Geometry check sheet. Reference: the model listing, model coordinates, mm. A direction names the side the tool comes from. Coordinates: 2 decimals unless noted, no trailing zeros. Loops run counter-clockwise (first coordinate to the right, second up) from the corner with the lowest first, then second, coordinate; pieces in that order, holes last. Notation, with made-up numbers: (-13.5, 48) -> (3.5, 48) arc R21 ccw to (3.5, 61) -> close; hole circle Ø8 at (28.25, -28.75). An arc over 180 degrees is marked (long way). Answer as a JSON object with one key per item and string values.
from build123d import *

# Parameters (mm, degrees)
SKETCH1_R           = 0.95
SKETCH1_R_2         = 2
SKETCH1_R_3         = 3
SKETCH1_R_4         = 1.047925013
SKETCH1_R_5         = 0.495
SKETCH1_R_6         = 0.65
BOSS_EXTRUDE1_DEPTH = 17.78
CUT_EXTRUDE1_DEPTH  = 14.78
BOSS_EXTRUDE2_DEPTH = 3
SKETCH4_W           = 10.78
SKETCH4_H           = 1.889736425
CUT_EXTRUDE2_DEPTH  = 2.5
SKETCH5_W           = 10.78
SKETCH5_H           = 1.889736425
BOSS_EXTRUDE3_DEPTH = 3
SKETCH6_R           = 0.8
BOSS_EXTRUDE4_DEPTH = 17.78


with BuildPart() as part:
    # Sketch1 → Boss-Extrude1 (new body)
    with BuildSketch(Plane.XY):
        with BuildLine():
            Line((35.5, 14.5), (34, 14.5))
            Line((34, 14.5), (31, 17.5))
            Line((31, 17.5), (30, 17.5))
            Line((30, 17.5), (30, -18))
            Line((30, -18), (30.2, -18))
            ThreePointArc((30.2, -18), (30.553553391, -18.146446609), (30.7, -18.5))
            Line((30.7, -18.5), (30.8, -18.5))
            Line((30.8, -18.5), (30.8, -16.8))
            Line((30.8, -16.8), (31.4, -15.3))
            Line((31.4, -15.3), (34.5875, -17.140303983))
            ThreePointArc((34.5875, -17.140303983), (35.136538106, -17.689342089), (35.3375, -18.439342089))
            Line((35.3375, -18.439342089), (35.5, -18.439342089))
            Line((35.5, -18.439342089), (35.5, -33.580082734))
            ThreePointArc((35.5, -33.580082734), (34.978350458, -34.92710906), (33.685520077, -35.57145972))
            Line((33.685520077, -35.57145972), (33.65, -35.610442716))
            Line((33.65, -35.610442716), (33.65, -40))
            Line((33.65, -40), (31.4, -40))
            Line((31.4, -40), (30.8, -39.4))
            Line((30.8, -39.4), (30.8, -36.374097914))
            Line((30.8, -36.374097914), (21, -39))
            Line((21, -39), (13, -39))
            ThreePointArc((13, -39), (12.707106781, -39.707106781), (12, -40))
            Line((12, -40), (-12, -40))
            ThreePointArc((-12, -40), (-13.414213562, -39.414213562), (-14, -38))
            Line((-14, -38), (-14, -22.5))
            Line((-14, -22.5), (-28, -22.5))
            ThreePointArc((-28, -22.5), (-29.414213562, -21.914213562), (-30, -20.5))
            Line((-30, -20.5), (-30, -3.828427125))
            Line((-30, -3.828427125), (-30.86027165, -2.830608771))
            Line((-30.86027165, -2.830608771), (-32.619050385, -0.790623261))
            ThreePointArc((-32.619050385, -0.790623261), (-33.80184622, 5.878164829), (-30, 11.483314774))
            Line((-30, 11.483314774), (-29.873, 11.483314774))
            Line((-29.873, 11.483314774), (-29.873, 20.5))
            Line((-29.873, 20.5), (-30, 20.5))
            ThreePointArc((-30, 20.5), (-29.414213562, 21.914213562), (-28, 22.5))
            Line((-28, 22.5), (-14, 22.5))
            Line((-14, 22.5), (-14, 38))
            ThreePointArc((-14, 38), (-13.414213562, 39.414213562), (-12, 40))
            Line((-12, 40), (12, 40))
            ThreePointArc((12, 40), (12.707106781, 39.707106781), (13, 39))
            Line((13, 39), (21, 39))
            Line((21, 39), (34.017568937, 35.512452349))
            ThreePointArc((34.017568937, 35.512452349), (35.086684889, 34.798133425), (35.5, 33.580582168))
            Line((35.5, 33.580582168), (35.5, 14.5))
        make_face()
        with Locations((32.4, 33.5)):
            Circle(SKETCH1_R, mode=Mode.SUBTRACT)
        with Locations((31.3, 28)):
            Circle(SKETCH1_R_2, mode=Mode.SUBTRACT)
        with Locations((24.5, -15.9)):
            Circle(SKETCH1_R_3, mode=Mode.SUBTRACT)
        with Locations((28.297263495, -29)):
            Circle(SKETCH1_R_4, mode=Mode.SUBTRACT)
        with Locations((28.297263495, -33)):
            Circle(SKETCH1_R_2, mode=Mode.SUBTRACT)
        with Locations((-26.5, -19.4)):
            Circle(SKETCH1_R_2, mode=Mode.SUBTRACT)
        with Locations((-9.958595339, -5.892279985)):
            Circle(SKETCH1_R_5, mode=Mode.SUBTRACT)
        with Locations((-32.65, 4)):
            Circle(SKETCH1_R_6, mode=Mode.SUBTRACT)
        with Locations((-26.5, 13.3)):
            Circle(SKETCH1_R, mode=Mode.SUBTRACT)
        with Locations((-26.5, 19.4)):
            Circle(SKETCH1_R_2, mode=Mode.SUBTRACT)
        with Locations((-20.3, 19.4)):
            Circle(SKETCH1_R_2, mode=Mode.SUBTRACT)
    extrude(amount=BOSS_EXTRUDE1_DEPTH)

    # Sketch2 → Cut-Extrude1 (cut)
    with BuildSketch(Plane.XY.offset(17.78)):
        with BuildLine():
            Line((-31.427876097, 11.660444431), (-29.178119463, 8.97928888))
            ThreePointArc((-29.178119463, 8.97928888), (-31.5, 4), (-29.178119463, -0.97928888))
            Line((-29.178119463, -0.97928888), (-31.427876097, -3.660444431))
            ThreePointArc((-31.427876097, -3.660444431), (-35, 4), (-31.427876097, 11.660444431))
        make_face()
    extrude(amount=-CUT_EXTRUDE1_DEPTH, mode=Mode.SUBTRACT)

    # Sketch3 → Boss-Extrude2 (add)
    with BuildSketch(Plane.XY.offset(17.78)):
        with BuildLine():
            Line((-29.178119463, -0.97928888), (-30.795044426, -2.906265014))
            ThreePointArc((-30.795044426, -2.906265014), (-34.015488692, 4), (-30.795044426, 10.906265014))
            Line((-30.795044426, 10.906265014), (-29.178119463, 8.97928888))
            ThreePointArc((-29.178119463, 8.97928888), (-31.5, 4), (-29.178119463, -0.97928888))
        make_face()
    extrude(amount=-BOSS_EXTRUDE2_DEPTH)

    # Sketch4 → Cut-Extrude2 (cut)
    with BuildSketch(Plane(origin=(-19.102021317, -16.468856625, 0), x_dir=(0, 0, 1), z_dir=(-0.757378649, -0.652975943, 0))):
        with Locations((8.89, 19.255785792)):
            Rectangle(SKETCH4_W, SKETCH4_H)
    extrude(amount=-CUT_EXTRUDE2_DEPTH, mode=Mode.SUBTRACT)

    # Sketch5 → Boss-Extrude3 (add)
    with BuildSketch(Plane(origin=(-17.208574695, -14.836416768, 0), x_dir=(0, 0, 1), z_dir=(-0.757378649, -0.652975943, 0))):
        with Locations((8.89, 19.255785792)):
            Rectangle(SKETCH5_W, SKETCH5_H)
    extrude(amount=BOSS_EXTRUDE3_DEPTH)

    # Sketch6 → Boss-Extrude4 (add)
    with BuildSketch(Plane.XY):
        with BuildLine():
            Line((-33.363800719, -0.692521635), (-30.744750334, -3.730325499))
            Line((-30.744750334, -3.730325499), (-33.186517311, -6.172092477))
            ThreePointArc((-33.186517311, -6.172092477), (-33.347465178, -6.279953339), (-33.53733329, -6.318531593))
            Line((-33.53733329, -6.318531593), (-35.164834129, -6.327442008))
            ThreePointArc((-35.164834129, -6.327442008), (-35.877415735, -6.034563776), (-36.170293967, -5.32198217))
            Line((-36.170293967, -5.32198217), (-36.161383552, -3.69448133))
            ThreePointArc((-36.161383552, -3.69448133), (-36.122805298, -3.504613219), (-36.014944436, -3.343665352))
            Line((-36.014944436, -3.343665352), (-33.363800719, -0.692521635))
        make_face()
        with Locations((-33.569032824, -3.517375453)):
            Circle(SKETCH6_R, mode=Mode.SUBTRACT)
    extrude(amount=BOSS_EXTRUDE4_DEPTH)


solid = part.part
1. Depth check by flat-ended pin: P1, Ø8, axis at y = -28, z = 12.5, coming from the -X side; P2, Ø5, axis at y = 18.5, z = 7.5, coming from the -X side; P3, Ø5, axis at y = -38.5, z = 8.5, coming from the +X side; P4, Ø2.5, axis at x = 28.3, y = -29, coming from the +Z side. Enter the tip coordinate at first touch or a pass-through.
Evaluation:
{"P1": "stops at x = -14", "P2": "stops at x = -30", "P3": "stops at x = 33.65", "P4": "stops at z = 17.78"}
2. Mould release check, pull along Z, two halves, no side actions. Record for faces 5 (the face through (-35, -4, 0)), 6 (the face through (35.5, -26, 9)), 7 (the face through (-31.362, 5.33, 8.972)): released by +Z, released by -Z, zero draft, split by the parting line, or undercut.
Evaluation:
{"face 5": "released by -Z", "face 6": "zero draft", "face 7": "undercut"}
3. Thickness scan on probe 1 along Y at (x, z) = (-26.5, 5.25); probe 2 along Y at (x, z) = (-20.3, 12); probe 3 along Y at (x, z) = (-26, 4.75). Record the ranges inside material, lowest first. Write a range as from..to.
Evaluation:
{"probe 1": "y = -22.5..-21.4, -17.4..12.35, 14.25..17.4, 21.4..22.5", "probe 2": "y = -22.5..17.4, 21.4..22.5", "probe 3": "y = -22.5..-21.34, -17.46..12.49, 14.11..17.46, 21.34..22.5"}
4. Section check B-B, the plane y = -29. Record the boundary of the cut face in (x, z).
Evaluation:
{"outline": "(-14, 0) -> (27.25, 0) -> (27.25, 17.78) -> (-14, 17.78) -> close; (29.35, 0) -> (35.5, 0) -> (35.5, 17.78) -> (29.35, 17.78) -> close"}
5. Section check A-A, the plane x = -20.3. Record the boundary of the cut face in (y, z), then the cut area to 3 significant figures.
Evaluation:
{"outline": "(-22.5, 0) -> (17.4, 0) -> (17.4, 17.78) -> (-22.5, 17.78) -> close; (21.4, 0) -> (22.5, 0) -> (22.5, 17.78) -> (21.4, 17.78) -> close", "area": "729 mm^2"}
6. Section check D-D, the plane y = 7. Record the boundary of the cut face in (x, z), then the cut area to 3 significant figures.
Evaluation:
{"outline": "(-33.5, 14.78) -> (-30.77, 14.78) -> (-30.77, 3) -> (-33.49, 3) -> (-33.49, 0) -> (30, 0) -> (30, 17.78) -> (-33.5, 17.78) -> close", "area": "1,100 mm^2"}
7. Tool access check on faces 1 (the face through (32.971, -16.207, 8.766)), 2 (the face through (-21, 22.5, 9)), 3 (the face through (-31.2, -3.2, 8.8)), 4 (the face through (-14, -30, 9)). Record the directions out of +Z, -Z, +X, -X, +Y, -Y that give a thin tool (end or side, any length) a straight path to the whole face; none if there is none.
Evaluation:
{"face 1": "+Z, -Z, +X", "face 2": "+Z, -Z, -X, +Y", "face 3": "none", "face 4": "+Z, -Z, -X, -Y"}
8. Section check C-C, the plane x = 32.4. Record the boundary of the cut face in (y, z), then the cut area to 3 significant figures.
Evaluation:
{"outline": "(-40, 0) -> (-15.88, 0) -> (-15.88, 17.78) -> (-40, 17.78) -> close; (16.1, 0) -> (26.33, 0) -> (26.33, 17.78) -> (16.1, 17.78) -> close; (29.67, 0) -> (32.55, 0) -> (32.55, 17.78) -> (29.67, 17.78) -> close; (34.45, 0) -> (35.95, 0) -> (35.95, 17.78) -> (34.45, 17.78) -> close", "area": "689 mm^2"}
